```python
from build123d import *

# Parameters (mm, degrees)
EXTRUDE_1_DEPTH        = 53
FILLET_1_R             = 8
F_16_0MM_1_D           = 14
F_16_0MM_1_CSINK_D     = 16.05
F_16_0MM_1_CSINK_ANGLE = 100
F_6_0MM_1_D            = 6
F_6_0MM_1_CSINK_D      = 6.05
F_6_0MM_1_CSINK_ANGLE  = 100
FILLET_4_R             = 8


with BuildPart() as part:
    # 草图2 → 凸台-拉伸1 (new body)
    with BuildSketch(Plane.XY):
        Polygon((0, 0), (53, 0), (53, 12), (-78.5, 12), (-78.5, 4), (-38.5, 4), align=None)
    extrude(amount=EXTRUDE_1_DEPTH)

    # 圆角1
    fillet_1_edges = [part.edges().sort_by_distance(p)[0] for p in [
        (53, 6, 0),
    ]]
    fillet(fillet_1_edges, radius=FILLET_1_R)

    # Ø16.0mm 暗销孔1 (through all)
    with Locations(Plane(origin=(0, 12, 0), x_dir=(1, 0, 0), z_dir=(0, 1, 0))):
        with Locations((26.5, -26.5)):
            CounterSinkHole(F_16_0MM_1_D / 2, F_16_0MM_1_CSINK_D / 2, counter_sink_angle=F_16_0MM_1_CSINK_ANGLE)

    # Ø6.0mm 暗销孔1 (through all)
    with Locations(Plane(origin=(0, 12, 0), x_dir=(1, 0, 0), z_dir=(0, 1, 0))):
        with Locations((-58.5, -25)):
            CounterSinkHole(F_6_0MM_1_D / 2, F_6_0MM_1_CSINK_D / 2, counter_sink_angle=F_6_0MM_1_CSINK_ANGLE)

    # 圆角4
    fillet_4_edges = [part.edges().sort_by_distance(p)[0] for p in [
        (53, 6, 53),
    ]]
    fillet(fillet_4_edges, radius=FILLET_4_R)


solid = part.part
```
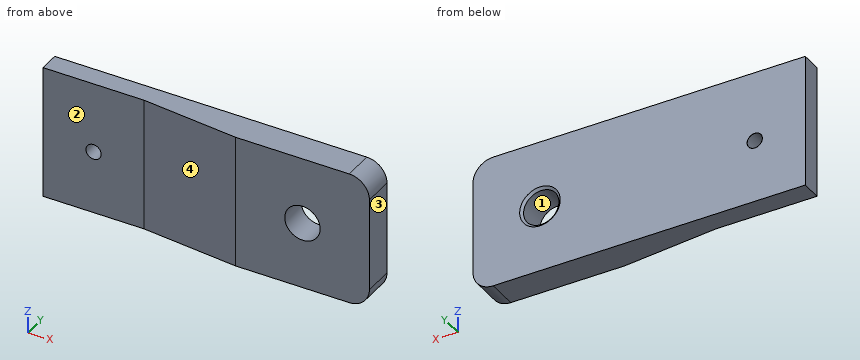
Part model, mm, in its own coordinate system. Face numbers are marked on the shaded views. Give positions to 0.01 mm unless a question says otherwise; leave off trailing zeros. Order: outer loops, then holes, each group sorted by start corner. A loop starts at its lowest first (then second) coordinate and runs counter-clockwise, first axis right, second up. Notation, with made-up numbers: M 35,-34.75 L 70,-34.75 A33 cw 70,0.25 Z; hole C 74.25,88.25 d5. An arc over 180 degrees is marked long. Use a Markdown table: item, result. Add a question column.
(1) Saw through at B-B, the plane y = 6.5. Give the cut face in (x, z), and give its area (3 significant figures).
(2) Drop a flat-ended pin along its axis: P1, Ø3, axis at x = -64.5, z = 9.5, coming from the -Y side. Give the stop position or say it passes through.
(3) Mould opens along X. For the marked faces 1, 2, 3 and 4 say: +X half, -X half, draft (parallel to the pull), parting line (faces both ways), or undercut.
(4) Saw through at D-D, the plane x = 26.5. Give the cut face in (y, z) (3 decimals), and give its area (3 significant figures).
(5) Saw through at C-C, the plane z = 36. Give the cut face in (x, y), and give its area (3 significant figures).
(6) Saw through at A-A, the plane x = -58.5. Give the cut face in (y, z) (3 decimals).
(7) Probe line 1 along X through (y, z) = (8.75, 26.5); line 2 along Y through (x, z) = (-66, 31); line 3 along X through (y, z) = (7.75, 24.5). List the from-to ranges inside material, lowest first. Write a range as [from, to].
Answer key:
| question | item | result |
|---|---|---|
| 1 | outline | M -78.5,0 L 45,0 A8 ccw 53,8 L 53,45 A8 ccw 45,53 L -78.5,53 Z; hole C -58.5,25 d6; hole C 26.5,26.5 d14 |
| 1 | area | 6,760 mm^2 |
| 2 | P1 | y = 4 |
| 3 | face 1 | undercut |
| 3 | face 2 | draft |
| 3 | face 3 | +X half |
| 3 | face 4 | -X half |
| 4 | outline | M 0,0 L 12,0 L 12,18.475 L 11.14,19.5 L 0,19.5 Z; M 0,33.5 L 11.14,33.5 L 12,34.525 L 12,53 L 0,53 Z |
| 4 | area | 467 mm^2 |
| 5 | outline | M -78.5,4 L -38.5,4 L 0,0 L 53,0 L 53,12 L -78.5,12 Z |
| 5 | area | 1,340 mm^2 |
| 6 | outline | M 4,0 L 12,0 L 12,21.975 L 11.979,22 L 4,22 Z; M 4,28 L 11.979,28 L 12,28.025 L 12,53 L 4,53 Z |
| 7 | line 1 | [-78.5, -61.1], [-55.9, 19.5], [33.5, 53] |
| 7 | line 2 | [4, 12] |
| 7 | line 3 | [-78.5, -61.46], [-55.54, 19.79], [33.21, 53] |
